Autodesk Inventor part; units mm, degrees
ref_plane "Начальная плоскость" through (0, 0, 0) normal (0, 0, 1) x (1, 0, 0)
ref_plane "Конечная плоскость" through (0, 0, 240.17) normal (0, 0, 1) x (1, 0, 0)
ref_plane "YZ Plane" through (0, 0, 0) normal (1, 0, 0) x (0, 1, 0)
ref_plane "Начальная плоскость" through (0, 0, 0) normal (0, 0, 1) x (1, 0, 0)
ref_plane "Конечная плоскость" through (0, 0, 240.17) normal (0, 0, 1) x (1, 0, 0)
sketch "Эскиз" plane through (0, 0, 0) normal (0, 0, 1) x (1, 0, 0)
  line L0 (-1.43, 0) -> (-1.43, 40)
  line L1 (-1.43, 40) -> (43.57, 40)
  line L2 (43.57, 40) -> (43.57, 38.1774)
  line L3 (39.9881, 34.1993) -> (11.2338, 31.1771)
  line L4 (4.07, 23.221) -> (4.07, 0)
  line L5 (4.07, 0) -> (-1.43, 0) construction
  line L6 (23.82, 40) -> (23.82, 32.5) construction
  line L7 (43.57, 34.5758) -> (43.57, 32.5) construction
  line L8 (43.57, 32.5) -> (23.82, 32.5) construction
  line L9 (0, 15) -> (0, -27) construction
  line L10 (-5.539, 0) -> (16.0067, 0) construction
  line L11 (-1.43, 0) -> (-1.43, -40)
  line L12 (-1.43, -40) -> (43.57, -40)
  line L13 (43.57, -40) -> (43.57, -38.1774)
  line L14 (39.9881, -34.1993) -> (11.2338, -31.1771)
  line L15 (4.07, -23.221) -> (4.07, 0)
  arc A0 (11.2338, 31.1771) -> (4.07, 23.221) centre (12.07, 23.221) ccw
  arc A1 (4.07, -23.221) -> (11.2338, -31.1771) centre (12.07, -23.221) ccw
  arc A2 (39.9881, 34.1993) -> (43.57, 38.1774) centre (39.57, 38.1774) ccw
  arc A3 (43.57, -38.1774) -> (39.9881, -34.1993) centre (39.57, -38.1774) ccw
  line L16 (0, 56) -> (0, -56) construction
  line L17 (-15.5135, 0) -> (54.308, 0) construction
  point P0 (4.07, 30.4242)
  point P1 (43.57, -34.5758)
  point P2 (4.07, -30.4242)
  point P3 (23.82, -40)
  point P4 (23.82, -32.5)
  dimension "d0" = 5.5
  dimension "d1" = 40
  dimension "d2" = 45
  dimension "d3" = 7.5
  dimension "d4" = 19.75
  dimension "d5" = 2.0758
  dimension "d23" = 8
  dimension "d24" = 4
  dimension "d25" = 1.43
extrude "Тело" add sketch "Эскиз" along normal up to surface (240.17 mm away) from surface at 0
sketch "Sketch3" plane through (0, 0, 0) normal (0, 0, 1) x (1, 0, 0)
  line L0 (0, 0) -> (10, 0)
ref_plane "Work Plane3" through (0, 0, 0) normal (0, -1, 0) x (1, 0, 0)
sketch "Sketch4" plane through (0, 0, 0) normal (0, -1, 0) x (1, 0, 0)
  line L0 (-2, 0) -> (12, 0)
  line L1 (-2, 240.17) -> (12, 240.17)
  dimension "d29" = 240.17
equation "\"d0\" = G_T"
equation "\"d1\" = 0.5 * G_H"
equation "\"d2\" = G_W"
equation "\"d3\" = G_T1"
equation "\"d4\" = G_C"
equation "\"d23\" = G_IR"
equation "\"d24\" = G_ER"
equation "\"d25\" = ex"
equation "\"d6\" = G_L"
equation "\"G_W\" = 45"
equation "\"G_T\" = 5.5"
equation "\"G_T1\" = 7.5"
equation "\"G_NG\" = 0.105104"
equation "\"G_ER\" = 4"
equation "\"G_IR\" = 8"
equation "\"G_C\" = 19.75"
equation "\"G_L\" = d29"
equation "\"ex\" = 1.43"
equation "\"G_OFFSET_START\" = 0"
equation "\"G_OFFSET_END\" = 0"
equation "\"d27\" = G_OFFSET_END + B_L"
equation "\"B_L\" = 240.17"
properties part number "ISO 657/11 - CH 80 x 8 - 240,17" material "Сталь, мягкая"
The listing builds one solid part. Answer for the finished solid, in the listing's coordinates (mm). A direction names the side the tool comes from. Give positions to 0.01 mm unless a question says otherwise; leave off trailing zeros. Loops run counter-clockwise (first coordinate to the right, second up) from the corner with the lowest first, then second, coordinate; pieces in that order, holes last. Notation, with made-up numbers: (37.5, -5.5) - (52.5, -5.5) arc R31 ccw to (52.5, 22.5) - close; hole circle Ø1 at (-27.75, 68.5). An arc over 180 degrees is marked (long way). Use one line per item in the form item = value.
1. Given pin 1 Ø5 at (y, z) = (10.5, 201.5) entering from +X; pin 2 Ø12 at (x, y) = (15.5, 9) entering from -Z, each flat-ended and moving along its own axis, determine where each tip first touches the part or whether it passes through.
Calculated:
pin_1 = 4.07
pin_2 = through
2. The mould has two halves that part along Y. Classify faces 3 (the face through (25.81, -32.71, 118.4)), 4 (the face through (21, 40, 118)), 5 (the face through (-1.43, -1, 118)): pulls with the +Y half, pulls with the -Y half, needs draft (parallel to the pull), parting line crosses it, or undercut.
Calculated:
face_3 = undercut
face_4 = pulls with the +Y half
face_5 = needs draft
3. Which of the six approach directions +Z, -Z, +X, -X, +Y, -Y give full straight-line access (tool end or side, diameter ignored) to faces 1 (the face through (6.07, 28.51, 118.4)), 2 (the face through (21, -40, 118))?
Calculated:
face_1 = +Z, -Z, +X
face_2 = +Z, -Z, +X, -X, -Y
4. Section C-C on y = 8.5 is taken. Give the vertices of the cut face in (x, z).
Calculated:
outline = (-1.43, 0) - (4.07, 0) - (4.07, 240.17) - (-1.43, 240.17) - close
5. Section A-A on x = 22 is taken. Give the vertices of the cut face in (y, z), then the cut area to 3 significant figures.
Calculated:
outline = (-40, 0) - (-32.31, 0) - (-32.31, 240.17) - (-40, 240.17) - close; (32.31, 0) - (40, 0) - (40, 240.17) - (32.31, 240.17) - close
area = 3,690 mm^2
6. Section B-B on z = 35.5 is taken. Give the vertices of the cut face in (x, y).
Calculated:
outline = (-1.43, -40) - (43.57, -40) - (43.57, -38.18) arc R4 ccw to (39.99, -34.2) - (11.23, -31.18) arc R8 cw to (4.07, -23.22) - (4.07, 23.22) arc R8 cw to (11.23, 31.18) - (39.99, 34.2) arc R4 ccw to (43.57, 38.18) - (43.57, 40) - (-1.43, 40) - close
7. Find the intervals of material crossed by line 1 along X through (y, z) = (16, 71.5); line 2 along Y through (x, z) = (34.5, 11); line 3 along Y through (x, z) = (9.5, 207.5), in increasing order. Write a range as [from, to].
Calculated:
line_1 = [-1.43, 4.07]
line_2 = [-40, -33.62], [33.62, 40]
line_3 = [-40, -30.8], [30.8, 40]
8. Section D-D on x = 7 is taken. Give the vertices of the cut face in (y, z), then the cut area to 3 significant figures.
Calculated:
outline = (-40, 0) - (-29.41, 0) - (-29.41, 240.17) - (-40, 240.17) - close; (29.41, 0) - (40, 0) - (40, 240.17) - (29.41, 240.17) - close
area = 5,090 mm^2
